Read the model definition and answer for the solid it produces. Units are mm, in the model's axes. Face numbers are marked on the shaded views. A direction names the side the tool comes from. Round coordinates to 2 decimals unless told otherwise and drop trailing zeros. Order: outer loops, then holes, each group sorted by start corner. A loop starts at its lowest first (then second) coordinate and runs counter-clockwise, first axis right, second up.
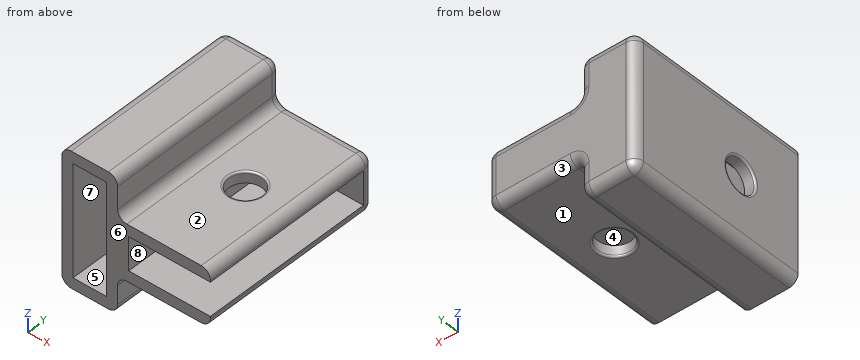
from build123d import *

# Parameters (mm, degrees)
BOSS_EXTRUDE1_DEPTH     = 100
SKETCH2_W               = 30
SKETCH2_H               = 100
BOSS_EXTRUDE3_DEPTH     = 50
SKETCH6_W               = 18
SKETCH6_H               = 94
CUT_EXTRUDE1_DEPTH      = 44
SKETCH7_W               = 18
SKETCH7_H               = 60
CUT_EXTRUDE2_DEPTH      = 94
SKETCH8_R               = 9
CUT_EXTRUDE3_DEPTH      = 1
CUT_EXTRUDE3_DEPTH_BACK = 81
FILLET1_R               = 5
SKETCH9_R               = 9
CUT_EXTRUDE4_DEPTH      = 51
FILLET2_R               = 1


with BuildPart() as part:
    # Sketch1 → Boss-Extrude1 (new body)
    with BuildSketch(Plane(origin=(0, 0, 0), x_dir=(1, 0, 0), z_dir=(0, 1, 0))):
        Polygon((24, 72), (30, 72), (30, 0), (0, 0), (0, 72), (6, 72), align=None)
    extrude(amount=BOSS_EXTRUDE1_DEPTH)

    # Sketch2 → Boss-Extrude3 (add)
    with BuildSketch(Plane(origin=(30, 0, 0), x_dir=(0, 0, -1), z_dir=(1, 0, 0))):
        with Locations((37, 50)):
            Rectangle(SKETCH2_W, SKETCH2_H)
    extrude(amount=BOSS_EXTRUDE3_DEPTH)

    # Sketch6 → Cut-Extrude1 (cut)
    with BuildSketch(Plane(origin=(80, 0, 0), x_dir=(0, 0, -1), z_dir=(1, 0, 0))):
        with Locations((37, 47)):
            Rectangle(SKETCH6_W, SKETCH6_H)
    extrude(amount=-CUT_EXTRUDE1_DEPTH, mode=Mode.SUBTRACT)

    # Sketch7 → Cut-Extrude2 (cut)
    with BuildSketch(Plane.XZ):
        with Locations((15, -36)):
            Rectangle(SKETCH7_W, SKETCH7_H)
    extrude(amount=-CUT_EXTRUDE2_DEPTH, mode=Mode.SUBTRACT)

    # Sketch8 → Cut-Extrude3 (cut, two sides)
    with BuildSketch(Plane.ZY) as cut_extrude3_sk:
        with Locations((-37, 35)):
            Circle(SKETCH8_R)
    extrude(amount=CUT_EXTRUDE3_DEPTH, mode=Mode.SUBTRACT)
    extrude(cut_extrude3_sk.sketch, amount=-CUT_EXTRUDE3_DEPTH_BACK, mode=Mode.SUBTRACT)

    # Fillet1
    fillet1_edges = [part.edges().sort_by_distance(p)[0] for p in [
        (30, 100, -11),
        (0, 50, -72),
        (30, 50, -72),
        (30, 50, 0),
        (0, 50, 0),
        (15, 100, -72),
        (30, 100, -62),
        (30, 50, -22),
        (55, 100, -22),
        (30, 50, -52),
        (55, 100, -52),
        (80, 50, -22),
        (80, 50, -52),
        (80, 100, -37),
        (0, 100, -36),
        (15, 100, 0),
    ]]
    fillet(fillet1_edges, radius=FILLET1_R)

    # Sketch9 → Cut-Extrude4 (cut, through all)
    with BuildSketch(Plane.XY.offset(-22)):
        with Locations((55, 50)):
            Circle(SKETCH9_R)
    extrude(amount=-CUT_EXTRUDE4_DEPTH, mode=Mode.SUBTRACT)

    # Fillet2
    fillet2_edges = [part.edges().sort_by_distance(p)[0] for p in [
        (46, 50, -52),
        (46, 50, -22),
        (0, 35, -46),
    ]]
    fillet(fillet2_edges, radius=FILLET2_R)


solid = part.part
Q1. A cutting plane is placed at B-B, the plane x = 55. Give the vertices of the cut face in (y, z), plus the area to 3 significant figures.
Outcome:
outline: (0, -52) - (40, -52) arc R1 ccw to (41, -51) - (41, -46) - (0, -46) - close; (0, -28) - (41, -28) - (41, -23) arc R1 ccw to (40, -22) - (0, -22) - close; (59, -51) arc R1 ccw to (60, -52) - (95, -52) arc R5 ccw to (100, -47) - (100, -27) arc R5 ccw to (95, -22) - (60, -22) arc R1 ccw to (59, -23) - (59, -28) - (94, -28) - (94, -46) - (59, -46) - close
area: 1,080 mm2
Q2. A cutting plane is placed at C-C, the plane z = -37. Give the vertices of the cut face in (x, y).
Outcome:
outline: (0, 0) - (6, 0) - (6, 26) - (1, 26) arc R1 ccw to (0, 25) - close; (0, 45) arc R1 ccw to (1, 44) - (6, 44) - (6, 94) - (24, 94) - (24, 44) - (36, 44) - (36, 94) - (80, 94) - (80, 95) arc R5 ccw to (75, 100) - (5, 100) arc R5 ccw to (0, 95) - close; (24, 0) - (36, 0) - (36, 26) - (24, 26) - close
Q3. A cutting plane is placed at A-A, the plane y = 9.5. Give the vertices of the cut face in (x, z), plus the area to 3 significant figures.
Outcome:
outline: (0, -67) arc R5 ccw to (5, -72) - (25, -72) arc R5 ccw to (30, -67) - (30, -57) arc R5 cw to (35, -52) - (75, -52) arc R5 ccw to (80, -47) - (80, -46) - (36, -46) - (36, -28) - (80, -28) - (80, -27) arc R5 ccw to (75, -22) - (35, -22) arc R5 cw to (30, -17) - (30, -5) arc R5 ccw to (25, 0) - (5, 0) arc R5 ccw to (0, -5) - close; hole (6, -66) - (24, -66) - (24, -6) - (6, -6) - close
area: 1,770 mm2
Q4. Flat-ended cylindrical pins translate along their axes: pin 1 (2 mm diameter, centred on x = 10, z = -33.5, fed in from -Y); pin 2 (5.5 mm diameter, centred on y = 69, z = -36, fed in from +X); pin 3 (10 mm diameter, centred on x = 50, z = -23.5, fed in from -Y); pin 4 (12 mm diameter, centred on x = 39.5, y = 88.5, fed in from -Z). Find the tip coordinate at first contact, or state that the pin passes through.
Outcome:
pin 1: stops at y = 94
pin 2: stops at x = 36
pin 3: stops at y = 0
pin 4: stops at z = -52.23
Q5. For a pull along X with two mould halves and no side action, classify the marked faces 6, 7 and 8 as released by +X, released by -X, zero draft, split by the parting line, or undercut.
Outcome:
face 6: zero draft
face 7: undercut
face 8: released by +X
Q6. Straight lines are drawn through the part: probe 1 along X at (y, z) = (27, -59); probe 2 along X at (y, z) = (89.5, -42); probe 3 along Z at (x, y) = (40, 7.5). For each, find the intervals that lie inside material, in ascending order.
Outcome:
probe 1: x = 0 to 6, 24 to 30
probe 2: x = 0 to 6, 24 to 36
probe 3: z = -52 to -46, -28 to -22
Q7. For the marked faces 1, 2, 3, 4 and 5, determine the directions among +Z, -Z, +X, -X, +Y, -Y from which every point of the face is accessible in a straight line to the end or side of a thin tool.
Outcome:
face 1: -Z, +X, +Y, -Y
face 2: +Z, +X, +Y, -Y
face 3: -Z, +X, +Y
face 4: +X, -Y
face 5: -Y
Q8. A cutting plane is placed at D-D, the plane x = 43.5. Give the vertices of the cut face in (y, z).
Outcome:
outline: (0, -52) - (95, -52) arc R5 ccw to (100, -47) - (100, -27) arc R5 ccw to (95, -22) - (0, -22) - (0, -28) - (94, -28) - (94, -46) - (0, -46) - close
